Geometry: final body of the model. Coordinates: model frame, mm. Round coordinates to 2 decimals unless told otherwise and drop trailing zeros. Write each loop counter-clockwise with the first axis right and the second up, starting at its lowest first coordinate (ties: lowest second). Pieces come first, ordered by that corner, then holes. Notation, with made-up numbers: (56.5, 78) -> (68.5, 78) arc R17 ccw to (68.5, 101) -> close; hole circle Ø3 at (-37, -18). An arc over 180 degrees is marked (long way). Use one line per item in the form item = value. Start each with the question number.
1. Pin query (flat end, axial travel): pin 1 Ø4 at (x, y) = (-4, -8.5) entering from -Z; pin 2 Ø6 at (x, z) = (5.5, 9) entering from +Y; pin 3 Ø3 at (x, z) = (2, 21.5) entering from -Y; pin 4 Ø3.5 at (x, y) = (0, -4) entering from +Z. Return the tip coordinate at first contact, or that it passes through.
2. Draft query along X for faces 1 (the face through (-11.32, -10.01, 5.73)), 2 (the face through (0, -2, 9)), 3 (the face through (0, 0, 20)). Return one class per face: pulls with the +X half, pulls with the -X half, needs draft (parallel to the pull), parting line crosses it, or undercut.
3. Line query: L1, parallel to X at y = -4, z = 7; L2, parallel to Z at x = -7.75, y = -2; L3, parallel to Y at x = 0, z = 9.25. Output: solid intervals per line, ascending.
4. Cut plane A-A, the plane y = -4. Return the cut outline in (x, z).
```python
from build123d import *

# Parameters (mm, degrees)
F0_W     = 27.7
F0_H     = 30
F1_DEPTH = 30
F5_DEPTH = 27.701
F6_R     = 2
F7_DEPTH = 30.001


with BuildPart() as f1:
    # F0 (on Top) → F1 (new body)
    with BuildSketch(Plane.XY):
        Rectangle(F0_W, F0_H)
    extrude(amount=F1_DEPTH)

    # F0 (on Top) → F4 section 0
    with BuildSketch(Plane.XY):
        with BuildLine():
            Line((-13.85, 15), (13.85, 15))
            ThreePointArc((13.85, 15), (0, 16), (-13.85, 15))
        make_face()
    # F3 (on face) → F4 section 1
    with BuildSketch(Plane.XY.offset(30)):
        with BuildLine():
            Line((-13.85, 15), (13.85, 15))
            ThreePointArc((13.85, 15), (0, 15.99788), (-13.85, 15))
        make_face()
    loft()

    # F2 (on face) → F5 (cut, through all)
    with BuildSketch(Plane.YZ.offset(13.85)):
        Polygon((-15, 5), (10, 30), (-15, 30), align=None)
    extrude(amount=-F5_DEPTH, mode=Mode.SUBTRACT)

    # F6 (on face) → F7 (cut, through all)
    with BuildSketch(Plane(origin=(0, 0, 0), x_dir=(1, 0, 0), z_dir=(0, 0, -1))):
        with Locations((0, 4)):
            Circle(F6_R)
        with BuildLine():
            Line((13.85, 5), (13.85, 15))
            Line((13.85, 15), (3.85, 15))
            ThreePointArc((3.85, 15), (10.164768, 11.314768), (13.85, 5))
        make_face()
        with BuildLine():
            Line((-13.85, 15), (-13.85, 5))
            ThreePointArc((-13.85, 5), (-10.164768, 11.314768), (-3.85, 15))
            Line((-3.85, 15), (-13.85, 15))
        make_face()
    extrude(amount=-F7_DEPTH, mode=Mode.SUBTRACT)


solid = f1.part
```
Outcome:
q1.pin_1 = 0
q1.pin_2 = 15.97
q1.pin_3 = 0
q1.pin_4 = through
q2.face_1 = pulls with the -X half
q2.face_2 = undercut
q2.face_3 = needs draft
q3.L1 = -13.85 to -2, 2 to 13.85
q3.L2 = 0 to 18
q3.L3 = -10.75 to -6, -2 to 16
q4.outline = (-13.85, 0) -> (-2, 0) -> (-2, 16) -> (-13.85, 16) -> close; (2, 0) -> (13.85, 0) -> (13.85, 16) -> (2, 16) -> close
